from build123d import *

# Parameters (mm, degrees)
RECTANGLE001_W   = 30
RECTANGLE001_H   = 7.5
EXTRUDE003_DEPTH = 30
SKETCH_R         = 3.2
EXTRUDE002_DEPTH = 15
EXTRUDE_DEPTH    = 10


with BuildPart() as extrude003:
    # Rectangle001 → Extrude003 (new body)
    with BuildSketch(Plane(origin=(-30, -3.75, -15), x_dir=(1, 0, 0), z_dir=(0, 0, 1))):
        with Locations((15, 3.75)):
            Rectangle(RECTANGLE001_W, RECTANGLE001_H)
    extrude(amount=EXTRUDE003_DEPTH)


with BuildPart() as extrude003_1:
    # Extrude003 placement: moved
    add(extrude003.part.moved(Location((-15, 0, -15))))


with BuildPart() as cut:
    # Sketch → Extrude002 (new body)
    with BuildSketch(Plane(origin=(-15, 0, -30), x_dir=(1, 0, 0), z_dir=(0, -1, 0))):
        with BuildLine():
            Line((-25.202842, 21.644358), (0, 30))
            Line((0, 30), (0, 0))
            Line((-25.202842, 8.355642), (0, 0))
            ThreePointArc((-25.202842, 21.644358), (-30, 15), (-25.202842, 8.355642))
        make_face()
        with Locations((-23, 15)):
            Circle(SKETCH_R, mode=Mode.SUBTRACT)
    extrude(amount=-EXTRUDE002_DEPTH)


with BuildPart() as cut_1:
    # Extrude002 placement: moved
    add(cut.part.moved(Location((0, -7.5, 0))))

    # Cut: cut Extrude003
    add(extrude003_1.part, mode=Mode.SUBTRACT)


with BuildPart() as body:
    # Sketch001 → Extrude (new body, symmetric)
    with BuildSketch(Plane.XZ):
        Polygon((-15, 0), (-15, 13), (-11, 13), (-11, -43), (-15, -43), (-15, -30), align=None)
    extrude(amount=EXTRUDE_DEPTH, both=True)

    # Fusion: union Cut
    add(cut_1.part)


solid = body.part
Check sheet for the modelled part. Datum: model origin and axes. Units: mm. A direction names the side the tool comes from. Coordinates: 2 decimals unless noted, no trailing zeros. Loops run counter-clockwise (first coordinate to the right, second up) from the corner with the lowest first, then second, coordinate; pieces in that order, holes last. Notation, with made-up numbers: (55, 83) -> (80, 83) arc R24 ccw to (80, 101) -> close; hole circle Ø3 at (-15.75, 12). An arc over 180 degrees is marked (long way). Write item = value, one per line. Start each with the question number.
1. Tool access check on faces 1 (the flat face through (-27, -3.75, -15)), 2 (the flat face through (-26, 7.5, -15)), 3 (the flat face through (-15, 0, -15)), 4 (the flat face through (-26, -7.5, -15)). Record the directions out of +Z, -Z, +X, -X, +Y, -Y that give a thin tool (end or side, any length) a straight path to the whole face; none if there is none.
2. Section check A-A on z = -15. Record the cut outline in (x, y).
3. Material ranges on line 1 (Y direction, x = -27.5, z = -19); line 2 (X direction, y = -6.25, z = -41); line 3 (Z direction, x = -38, y = -6.25), recorded low to high.
4. Section check D-D on y = -0.5. Record the cut outline in (x, z), then the cut area to 3 significant figures.
5. Section check C-C on x = -38. Record the cut outline in (y, z).
6. Depth check by flat-ended pin: P1, Ø8.5, axis at x = -38, z = -15, coming from the +Y side; P2, Ø4, axis at x = -32, z = -10.5, coming from the -Y side; P3, Ø1.5, axis at y = 2, z = -20.5, coming from the -X side. Enter the tip coordinate at first touch or a pass-through.
7. Draft check along Z on faces 5 (the flat face through (-27.778, -5.651, -25.764)), 6 (the flat face through (-13, -10, -15)), 7 (the cylindrical face through (-40.539, 5.599, -16.947)). Enter one of: released by +Z, released by -Z, zero draft, split by the parting line, or undercut.
8. Section check B-B on x = -21.5. Record the cut outline in (y, z), then the cut area to 3 significant figures.
Responses:
q1.face_1 = +Z, -Z, -X
q1.face_2 = +Z, -Z, -X, +Y
q1.face_3 = -X
q1.face_4 = +Z, -Z, -X, -Y
q2.outline = (-45, -7.5) -> (-41.2, -7.5) -> (-41.2, -3.75) -> (-45, -3.75) -> close; (-45, 3.75) -> (-41.2, 3.75) -> (-41.2, 7.5) -> (-45, 7.5) -> close; (-34.8, -7.5) -> (-15, -7.5) -> (-15, -10) -> (-11, -10) -> (-11, 10) -> (-15, 10) -> (-15, 7.5) -> (-34.8, 7.5) -> (-34.8, 3.75) -> (-15, 3.75) -> (-15, -3.75) -> (-34.8, -3.75) -> close
q3.line_1 = -7.5 to -3.75, 3.75 to 7.5
q3.line_2 = -15 to -11
q3.line_3 = -22.37 to -18.2, -11.8 to -7.63
q4.outline = (-15, -43) -> (-11, -43) -> (-11, 13) -> (-15, 13) -> close
q4.area = 224 mm2
q5.outline = (-7.5, -22.37) -> (-3.75, -22.37) -> (-3.75, -18.2) -> (-7.5, -18.2) -> close; (-7.5, -11.8) -> (-3.75, -11.8) -> (-3.75, -7.63) -> (-7.5, -7.63) -> close; (3.75, -22.37) -> (7.5, -22.37) -> (7.5, -18.2) -> (3.75, -18.2) -> close; (3.75, -11.8) -> (7.5, -11.8) -> (7.5, -7.63) -> (3.75, -7.63) -> close
q6.P1 = 7.5
q6.P2 = -7.5
q6.P3 = -15
q7.face_5 = released by -Z
q7.face_6 = zero draft
q7.face_7 = undercut
q8.outline = (-7.5, -27.85) -> (-3.75, -27.85) -> (-3.75, -2.15) -> (-7.5, -2.15) -> close; (3.75, -27.85) -> (7.5, -27.85) -> (7.5, -2.15) -> (3.75, -2.15) -> close
q8.area = 193 mm2
